from build123d import *

# Parameters (mm, degrees)
SKETCH1_W           = 171.45
SKETCH1_H           = 36.83
BOSS_EXTRUDE1_DEPTH = 3.175
SKETCH2_W           = 12.7
SKETCH2_H           = 3.175
SKETCH2_W_2         = 50.8
BOSS_EXTRUDE2_DEPTH = 3.175
SKETCH3_W           = 42.418
SKETCH3_H           = 12.7
CUT_EXTRUDE1_DEPTH  = 3.175
SKETCH5_W           = 17.018
SKETCH5_H           = 12.7
BOSS_EXTRUDE3_DEPTH = 3.175
SKETCH6_W           = 3.175
SKETCH6_H           = 17.78
BOSS_EXTRUDE4_DEPTH = 3.175


with BuildPart() as part:
    # Sketch1 → Boss-Extrude1 (new body)
    with BuildSketch(Plane(origin=(0, 0, 0), x_dir=(1, 0, 0), z_dir=(0, 1, 0))):
        with Locations((85.725, 18.415)):
            Rectangle(SKETCH1_W, SKETCH1_H)
    extrude(amount=BOSS_EXTRUDE1_DEPTH)

    # Sketch2 → Boss-Extrude2 (add)
    with BuildSketch(Plane(origin=(0, 3.175, 0), x_dir=(1, 0, 0), z_dir=(0, 1, 0))):
        with Locations((15.875, -1.5875)):
            Rectangle(SKETCH2_W, SKETCH2_H)
        with Locations((41.275, -1.5875)):
            Rectangle(SKETCH2_W, SKETCH2_H)
        with Locations((85.725, -1.5875)):
            Rectangle(SKETCH2_W_2, SKETCH2_H)
        with Locations((130.175, -1.5875)):
            Rectangle(SKETCH2_W, SKETCH2_H)
        with Locations((155.575, -1.5875)):
            Rectangle(SKETCH2_W, SKETCH2_H)
    boss_extrude2 = extrude(amount=-BOSS_EXTRUDE2_DEPTH)

    # Sketch3 → Cut-Extrude1 (cut)
    with BuildSketch(Plane(origin=(0, 3.175, 0), x_dir=(1, 0, 0), z_dir=(0, 1, 0))):
        with Locations((88.646, 9.525)):
            Rectangle(SKETCH3_W, SKETCH3_H)
    extrude(amount=-CUT_EXTRUDE1_DEPTH, mode=Mode.SUBTRACT)

    # Sketch5 → Boss-Extrude3 (add)
    with BuildSketch(Plane(origin=(0, 3.175, 0), x_dir=(1, 0, 0), z_dir=(0, 1, 0))):
        with Locations((89.916, 9.525)):
            Rectangle(SKETCH5_W, SKETCH5_H)
    extrude(amount=-BOSS_EXTRUDE3_DEPTH)

    # Sketch6 → Boss-Extrude4 (add)
    with BuildSketch(Plane(origin=(0, 3.175, 0), x_dir=(1, 0, 0), z_dir=(0, 1, 0))):
        with Locations((-1.5875, 18.415)):
            Rectangle(SKETCH6_W, SKETCH6_H)
        with Locations((173.0375, 18.415)):
            Rectangle(SKETCH6_W, SKETCH6_H)
    extrude(amount=-BOSS_EXTRUDE4_DEPTH)

    # Mirror1: Boss-Extrude2 across plane
    add(boss_extrude2.mirror(Plane(origin=(0, 0, -18.415), x_dir=(1, 0, 0), z_dir=(0, 0, -1))))


solid = part.part
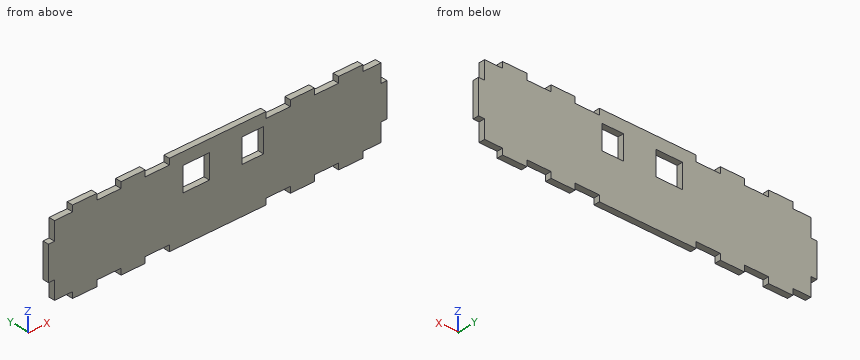
Can you work these out from the model? Positions are in its coordinate system, mm. Coordinates: 2 decimals unless noted, no trailing zeros. Write each loop counter-clockwise with the first axis right and the second up, starting at its lowest first coordinate (ties: lowest second). Pieces come first, ordered by that corner, then holes. Notation, with made-up numbers: (24.5, 87.25) -> (75.5, 87.25) arc R25 ccw to (75.5, 114.25) -> close; hole circle Ø3 at (-2.75, -17). An arc over 180 degrees is marked (long way). Write each question's results on one line, items separated by ' | '. Start each with the question number.
Item 1: If we section it at C-C, the plane y = 1.45: Count the separate pieces of the cut face and the enclosed holes in it, and give its area (3 significant figures).
Item 2: Please list where these lines run through material, in increasing order: probe 1 along X at (y, z) = (1.8, -37) (3 decimals); probe 2 along X at (y, z) = (2.3, -9) (3 decimals); probe 3 along X at (y, z) = (0.65, -14) (3 decimals).
Item 3: If we section it at B-B, the plane z = -13: Write out the boundary of the cut face in (x, y) (3 decimals).
Item 4: I'm going to push flat-ended pins straight in: P1, Ø1, axis at x = 167, y = 1.5, coming from the +Z side; P2, Ø1.6, axis at x = 4.5, y = 1.5, coming from the -Z side; P3, Ø1, axis at y = 1, z = -39, coming from the -X side (3 decimals). Where does each tip first touch, or does it pass through?
Item 5: If we section it at A-A, the plane x = 100: Write out the boundary of the cut face in (y, z) (3 decimals), and give its area (3 significant figures).
Item 6: If we section it at D-D, the plane z = -6: Write out the boundary of the cut face in (x, y) (3 decimals).
Answer block:
1) separate pieces: 1 | enclosed holes: 2 | area: 6,750 mm²
2) probe 1: 9.525 to 22.225, 34.925 to 47.625, 60.325 to 111.125, 123.825 to 136.525, 149.225 to 161.925 | probe 2: 0 to 67.437, 81.407 to 98.425, 109.855 to 171.45 | probe 3: -3.175 to 67.437, 81.407 to 98.425, 109.855 to 174.625
3) outline: (-3.175, 0) -> (67.437, 0) -> (67.437, 3.175) -> (-3.175, 3.175) -> close; (81.407, 0) -> (98.425, 0) -> (98.425, 3.175) -> (81.407, 3.175) -> close; (109.855, 0) -> (174.625, 0) -> (174.625, 3.175) -> (109.855, 3.175) -> close
4) P1: z = 0 | P2: z = -36.83 | P3: x = 9.525
5) outline: (0, -40.005) -> (3.175, -40.005) -> (3.175, -15.875) -> (0, -15.875) -> close; (0, -3.175) -> (3.175, -3.175) -> (3.175, 3.175) -> (0, 3.175) -> close | area: 96.8 mm²
6) outline: (0, 0) -> (67.437, 0) -> (67.437, 3.175) -> (0, 3.175) -> close; (81.407, 0) -> (98.425, 0) -> (98.425, 3.175) -> (81.407, 3.175) -> close; (109.855, 0) -> (171.45, 0) -> (171.45, 3.175) -> (109.855, 3.175) -> close
